Could you check a few things on this model? Use its own coordinates, in mm. Face numbers are marked on the shaded views. A direction names the side the tool comes from. Give positions to 0.01 mm unless a question says otherwise; leave off trailing zeros. Write each loop counter-clockwise with the first axis right and the second up, starting at its lowest first coordinate (ties: lowest second). Pieces come first, ordered by that corner, then holes. Notation, with made-up numbers: (33.5, 76.25) - (70.5, 76.25) arc R32 ccw to (70.5, 113.25) - close; hole circle Ø8 at (30.25, 73.5). An arc over 180 degrees is marked (long way). Answer as CSV lines item,"result". Start each with the question number.
Q1. Imagine slicing it at D-D on z = 29. List the corners of the cut face in (x, y) for me.
Q2. Imagine slicing it at B-B on y = 12.5. List the corners of the cut face in (x, z) for me, and give its area (3 significant figures).
Q3. Will these pins go through, and if not, where does the flat tip stop? pin 1 Ø2 at (y, z) = (11.5, 25.5) entering from +X; pin 2 Ø2.5 at (x, z) = (12.5, 68) entering from +Y; pin 3 Ø1.6 at (y, z) = (12.5, 68) entering from +X.
Q4. If I drill on line 1 along Z through (x, y) = (3.95, 12.5); line 2 along Y through (x, z) = (3.55, 12); line 3 along X through (y, z) = (12.5, 26.5), over which ranges is the centre line in solid material (lowest first)?
Q5. On a 3-axis mill with a long thin cutter (end or side, diameter ignored), from which of +Z, -Z, +X, -X, +Y, -Y can I reach the whole of each face in a straight line? I mean the marked faces 1 and 2. Say none if no direction works.
Q6. Imagine slicing it at A-A on z = 12. List the corners of the cut face in (x, y) for me, and give its area (3 significant figures).
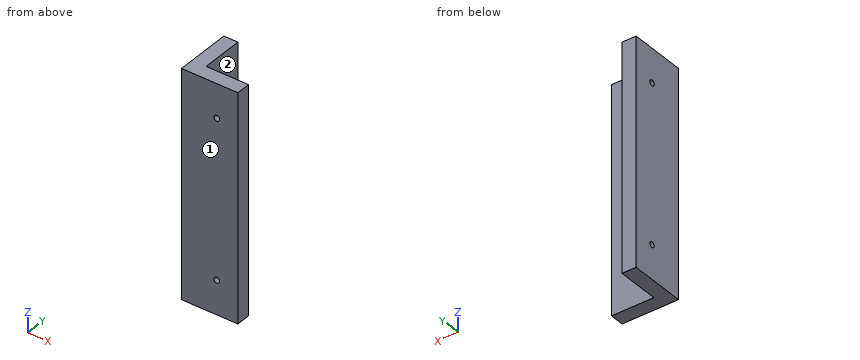
```python
from build123d import *

# Parameters (mm, degrees)
EXTRUDE_1_DEPTH          = 80
SKETCH_2_R               = 1
CUT_EXTRUDE_2_DEPTH      = 10
CUT_EXTRUDE_2_DEPTH_BACK = 10
SKETCH_3_R               = 1
CUT_EXTRUDE_3_DEPTH      = 10
CUT_EXTRUDE_3_DEPTH_BACK = 10


with BuildPart() as part:
    # 草圖1 → 填料-伸長1 (new body)
    with BuildSketch(Plane.XY):
        Polygon((0, 0), (0, 20), (5, 20), (5, 5), (20, 5), (20, 0), align=None)
    extrude(amount=EXTRUDE_1_DEPTH)

    # 草圖2 → 除料-伸長2 (cut, two sides)
    with BuildSketch(Plane(origin=(0, 0, 0), x_dir=(1, 0, 0), z_dir=(0, 1, 0))) as cut_extrude_2_sk:
        with Locations((12.5, -12)):
            Circle(SKETCH_2_R)
        with Locations((12.5, -68)):
            Circle(SKETCH_2_R)
    extrude(amount=CUT_EXTRUDE_2_DEPTH, mode=Mode.SUBTRACT)
    extrude(cut_extrude_2_sk.sketch, amount=-CUT_EXTRUDE_2_DEPTH_BACK, mode=Mode.SUBTRACT)

    # 草圖3 → 除料-伸長3 (cut, two sides)
    with BuildSketch(Plane(origin=(0, 0, 0), x_dir=(0, 0, -1), z_dir=(1, 0, 0))) as cut_extrude_3_sk:
        with Locations((-12, 12.5)):
            Circle(SKETCH_3_R)
        with Locations((-68, 12.5)):
            Circle(SKETCH_3_R)
    extrude(amount=CUT_EXTRUDE_3_DEPTH, mode=Mode.SUBTRACT)
    extrude(cut_extrude_3_sk.sketch, amount=-CUT_EXTRUDE_3_DEPTH_BACK, mode=Mode.SUBTRACT)


solid = part.part
```
Conclusion:
1,outline,"(0, 0) - (20, 0) - (20, 5) - (5, 5) - (5, 20) - (0, 20) - close"
2,outline,"(0, 0) - (5, 0) - (5, 11) - (0, 11) - close; (0, 13) - (5, 13) - (5, 67) - (0, 67) - close; (0, 69) - (5, 69) - (5, 80) - (0, 80) - close"
2,area,"380 mm^2"
3,pin 1,"x = 5"
3,pin 2,"y = 5"
3,pin 3,"through"
4,line 1,"0 to 11, 13 to 67, 69 to 80"
4,line 2,"0 to 11.5, 13.5 to 20"
4,line 3,"0 to 5"
5,face 1,"+Z, -Z, +X, -X, -Y"
5,face 2,"+Z, -Z, +X, +Y"
6,outline,"(0, 0) - (11.5, 0) - (11.5, 5) - (5, 5) - (5, 11.5) - (0, 11.5) - close; (0, 13.5) - (5, 13.5) - (5, 20) - (0, 20) - close; (13.5, 0) - (20, 0) - (20, 5) - (13.5, 5) - close"
6,area,"155 mm^2"
